Input: part model. Units: mm. Frame: model coordinates. A direction names the side the tool comes from. Coordinates: 2 decimals unless noted, no trailing zeros. Loops run counter-clockwise (first coordinate to the right, second up) from the corner with the lowest first, then second, coordinate; pieces in that order, holes last.
Item 1: Section C-C on z = 5. Return loops of the section in (x, y), and give its area (3 significant figures).
Item 2: Section D-D on z = -1. Give the number of separate pieces and of enclosed holes in the cut face, and give its area (3 significant figures).
Item 3: Reachability of faces 1 (the flat face through (-3, 8, -6)), 2 (the cylindrical face through (-7.8, -5.42, 5.42)), 3 (the cylindrical face through (-2.422, 3.075, -2.168)), 4 (the cylindrical face through (0.3, 3.4, 3.1)) from +Z, -Z, +X, -X, +Y, -Y: full face, straight path, thin tool, end or side. Return the list, or none.
Item 4: Contact query for flat-ended pins moving along their axis: P1, Ø10, axis at x = 1, y = -0.5, coming from the +Z side; P2, Ø3.5, axis at x = 12, y = 12, coming from the -Z side; P3, Ø1.2, axis at y = 8, z = -6, coming from the +X side. Output: stop coordinate, or through.
Item 5: Section B-B on y = 11. Return loops of the section in (x, z).
Item 6: Ray query, line 1 along Y through (x, z) = (0, -2.25); line 2 along Y through (x, z) = (0, 3.1); line 3 along X through (y, z) = (-6, -1). Return the intervals inside material, ascending.
Item 7: Section A-A on x = -12. Return loops of the section in (y, z).
Autodesk Inventor part; units mm, degrees
ref_plane "YZ Plane" through (0, 0, 0) normal (1, 0, 0) x (0, 1, 0)
ref_plane "XZ Plane" through (0, 0, 0) normal (0, 1, 0) x (-1, 0, 0)
ref_plane "XY Plane" through (0, 0, 0) normal (0, 0, 1) x (1, 0, 0)
sketch "Sketch1" plane through (0, 0, 0) normal (0, 0, 1) x (1, 0, 0)
  line L0 (15, 15) -> (-15, 15)
  line L1 (-15, 15) -> (-15, -15)
  line L2 (-15, -15) -> (15, -15)
  line L3 (15, -15) -> (15, 15)
  point P0 (0, 0)
  point P1 (15, 0)
  point P2 (0, 15)
  dimension "d0" = 30
extrude "Extrusion1" add sketch "Sketch1" along normal blind 2.3876
fillet "Fillet1" radius 5 4 edges at (15, 15, 1.1938) (-15, 15, 1.1938) (-15, -15, 1.1938) (15, -15, 1.1938)
sketch "Sketch2" plane through (0, 0, 2.3876) normal (0, 0, 1) x (1, 0, 0)
  line L0 (10, -15) -> (-10, -15)
  line L1 (15, 10) -> (15, -10)
  line L2 (-10, 15) -> (10, 15)
  line L3 (-15, -10) -> (-15, 10)
  point P0 (-12, 12)
  point P1 (12, 12)
  point P2 (12, -12)
  point P3 (-12, -12)
  dimension "d4" = 3
  dimension "d5" = 3
  dimension "d6" = 3
  dimension "d7" = 3
hole "Hole1" at (-12, 12, 2.3876) at (12, 12, 2.3876) at (12, -12, 2.3876) at (-12, -12, 2.3876) direction (0, 0, -1) diameter 3 end through all
sketch "Sketch3" plane through (0, 0, 2.3876) normal (0, 0, 1) x (1, 0, 0)
  line L0 (15, 10) -> (15, -10)
  line L1 (-10, 15) -> (10, 15)
  circle A0 centre (0, 0) radius 12.5
  point P0 (15, 0)
  point P1 (0, 15)
  dimension "d15" = 25
extrude "Extrusion2" add sketch "Sketch3" along normal blind 5
sketch "Sketch4" plane through (0, 0, 7.3876) normal (0, 0, 1) x (1, 0, 0)
  circle A0 centre (0, 0) radius 12.5
  circle A1 centre (0, 0) radius 9.5
  dimension "d86" = 3
extrude "Extrusion3" cut sketch "Sketch4" against normal blind 4 contours A1
sketch "Sketch5" plane through (0, 0, 7.3876) normal (0, 0, 1) x (1, 0, 0)
  circle A0 centre (0, 0) radius 9.5
  circle A1 centre (0, 0) radius 12.5
  circle A2 centre (0, 0) radius 10.5
  line L0 (-2, 9.2871) -> (-2, 10.3078)
  line L1 (2, 9.2871) -> (2, 10.3078)
  dimension "d23" = 4
  dimension "d85" = 2
extrude "Extrusion4" cut sketch "Sketch5" against normal up to surface (4 mm away) contours A0 L0 A2 L1 picked at (-1.557, 9.6904)
sketch "Sketch6" plane through (0, 0, 7.3876) normal (0, 0, 1) x (1, 0, 0)
  line L0 (2, 10.3078) -> (2, 9.2871)
  arc A0 (-2, 9.2871) -> (2, 9.2871) centre (0, 0) ccw
  line L1 (-2, 9.2871) -> (-2, 10.3078)
  arc A1 (2, 10.3078) -> (-2, 10.3078) centre (0, 0) ccw
  circle A2 centre (0, 0) radius 12.5
  circle A3 centre (0, 0) radius 10.5
  line L2 (-9.3841, -1.4792) -> (-10.3549, -1.7393)
  line L3 (-8.8665, -3.411) -> (-9.8373, -3.6712)
  line L4 (-6.2379, -7.1651) -> (-6.8143, -7.9884)
  line L5 (-5.176, -9.1356) -> (-4.5996, -8.3123)
  line L6 (4.5996, -8.3123) -> (5.176, -9.1356)
  line L7 (6.2379, -7.1651) -> (6.8143, -7.9884)
  line L8 (9.4984, 0.1728) -> (10.4997, 0.0852)
  line L9 (9.3241, -1.8196) -> (10.3253, -1.9072)
  dimension "d26" = 105
  dimension "d27" = 2
  dimension "d30" = 2
  dimension "d31" = 40
  dimension "d32" = 70
  dimension "d33" = 2
  dimension "d34" = 2
  dimension "d35" = 50
extrude "Extrusion5" cut sketch "Sketch6" against normal up to surface (4 mm away) contours L0 A0 L1 A1 | A3 L9 A0 L8 | L2 A0 L3 A3 | L7 A3 L6 A0 | L4 A0 L5 A3
sketch "Sketch7" plane through (0, 0, 3.3876) normal (0, 0, 1) x (1, 0, 0)
  arc A0 (2, 10.3078) -> (-2, 10.3078) centre (0, 0) ccw
  circle A1 centre (0, 0) radius 8
  arc A2 (-2, 9.2871) -> (-9.3841, -1.4792) centre (0, 0) ccw
  dimension "d84" = 1.5
extrude "Extrusion6" add sketch "Sketch7" along normal blind 0.381
sketch "Sketch8" plane through (0, 0, 0) normal (0, 0, -1) x (-1, 0, 0)
  line L0 (-10, 15) -> (10, 15)
  line L1 (-15, -10) -> (-15, 10)
  circle A0 centre (0, 0) radius 10
  point P0 (-15, 0)
  point P1 (0, 15)
  dimension "d39" = 20
extrude "Extrusion7" add sketch "Sketch8" along normal blind 5.715
sketch "Sketch9" plane through (0, 0, -5.715) normal (0, 0, -1) x (-1, 0, 0)
  circle A0 centre (0, 0) radius 10
  circle A1 centre (0, 0) radius 9
  dimension "d83" = 1
extrude "Extrusion8" add sketch "Sketch9" along normal blind 1.27 contours A1
sketch "Sketch10" plane through (0, 0, -6.985) normal (0, 0, -1) x (-1, 0, 0)
  circle A0 centre (0, 0) radius 9
  circle A1 centre (0, 0) radius 8
  line L0 (-3, 7.4162) -> (-3, 8.4853)
  line L1 (3, 7.4162) -> (3, 8.4853)
  dimension "d46" = 6
  dimension "d82" = 1
extrude "Extrusion9" cut sketch "Sketch10" against normal up to surface (1.27 mm away) contours L1 A1 L0 A0 picked at (-1.8485, 8.4268)
sketch "Sketch11" plane through (0, 0, 3.7686) normal (0, 0, 1) x (1, 0, 0)
  circle A0 centre (0, 0) radius 8
  line L0 (0, 0) -> (0, 6) construction
  point P0 (0, 3)
  point P1 (-2.1213, 2.1213)
  point P2 (-3, 0)
  point P3 (-2.1213, -2.1213)
  point P4 (0, -3)
  point P5 (2.1213, -2.1213)
  point P6 (3, 0)
  point P7 (2.1213, 2.1213)
  point P8 (4.2426, 4.2426)
  point P9 (6, 0)
  point P10 (4.2426, -4.2426)
  point P11 (0, -6)
  point P12 (-4.2426, -4.2426)
  point P13 (-6, 0)
  point P14 (-4.2426, 4.2426)
  dimension "d49" = 3
  dimension "d52" = 360
  dimension "d87" = 6
  dimension "d90" = 360
hole "Hole2" at (0, 0, 3.7686) at (0, 3, 3.7686) at (-2.1213, 2.1213, 3.7686) at (-3, 0, 3.7686) at (-2.1213, -2.1213, 3.7686) at (0, -3, 3.7686) at (2.1213, -2.1213, 3.7686) at (3, 0, 3.7686) at (2.1213, 2.1213, 3.7686) at (0, 6, 3.7686) at (4.2426, 4.2426, 3.7686) at (6, 0, 3.7686) at (4.2426, -4.2426, 3.7686) at (0, -6, 3.7686) at (-4.2426, -4.2426, 3.7686) at (-6, 0, 3.7686) at (-4.2426, 4.2426, 3.7686) direction (0, 0, -1) diameter 1 end through all
sketch "Sketch12" plane through (0, 0, -6.985) normal (0, 0, -1) x (-1, 0, 0)
  circle A0 centre (-3, 0) radius 0.5
  circle A1 centre (0, -3) radius 0.5
  circle A2 centre (3, 0) radius 0.5
  circle A3 centre (0, 3) radius 0.5
  circle A4 centre (0, 0) radius 0.5
  circle A5 centre (2.1213, 2.1213) radius 0.5
  circle A6 centre (2.1213, -2.1213) radius 0.5
  circle A7 centre (-2.1213, -2.1213) radius 0.5
  circle A8 centre (-2.1213, 2.1213) radius 0.5
  point P0 (6, 0)
  point P1 (0, -6)
  point P2 (-6, 0)
  point P3 (0, 6)
  point P4 (-4.2426, 4.2426)
  point P5 (-4.2426, -4.2426)
  point P6 (4.2426, -4.2426)
  point P7 (4.2426, 4.2426)
  point P8 (0, 0)
  point P9 (0, 0)
hole "Hole3" at (0, 3, -6.985) at (2.1213, 2.1213, -6.985) at (3, 0, -6.985) at (2.1213, -2.1213, -6.985) at (0, 0, -6.985) at (-2.1213, 2.1213, -6.985) at (-3, 0, -6.985) at (-2.1213, -2.1213, -6.985) at (0, -3, -6.985) at (4.2426, 4.2426, -6.985) at (0, 6, -6.985) at (-4.2426, 4.2426, -6.985) at (-6, 0, -6.985) at (-4.2426, -4.2426, -6.985) at (0, -6, -6.985) at (4.2426, -4.2426, -6.985) at (6, 0, -6.985) direction (0, 0, 1) diameter 2 depth 9.5
sketch "Sketch13" plane through (0, 0, -6.985) normal (0, 0, -1) x (-1, 0, 0)
  arc A0 (-3, 8.4853) -> (3, 8.4853) centre (0, 0) ccw
  line L0 (3, 8.4853) -> (3, 7.4162)
  arc A1 (3, 7.4162) -> (-3, 7.4162) centre (0, 0) ccw
  circle A2 centre (0, 0) radius 8
  line L1 (-2.5, -8.6458) -> (-2.5, -7.5993)
  line L2 (2.5, -8.6458) -> (2.5, -7.5993)
  dimension "d68" = 5
extrude "Extrusion10" cut sketch "Sketch13" against normal up to surface (1.27 mm away) contours L1 A2 L2 A0
sketch "Sketch25" plane through (0, 0, 3.7686) normal (0, 0, 1) x (1, 0, 0)
  line L0 (-1.0163, 4.6819) -> (0.1279, 4.6819) construction
  line L1 (0.1279, 4.6819) -> (0.1279, 3.2031) construction
  line L2 (0.1279, 3.2031) -> (-1.0163, 3.2031) construction
  line L3 (-1.0163, 3.2031) -> (-1.0163, 4.6819) construction
  line L4 (3.2538, -0.055) -> (3.2538, 1.4238) construction
  line L5 (3.2538, 1.4238) -> (4.398, 1.4238) construction
  line L6 (4.398, 1.4238) -> (4.398, -0.055) construction
  line L7 (4.398, -0.055) -> (3.2538, -0.055) construction
  line L8 (1.6906, 2.4904) -> (1.6906, 3.9692) construction
  line L9 (1.6906, 3.9692) -> (2.8348, 3.9692) construction
  line L10 (2.8348, 3.9692) -> (2.8348, 2.4904) construction
  line L11 (2.8348, 2.4904) -> (1.6906, 2.4904) construction
  line L12 (-2.7944, -4.281) -> (-2.7944, -2.8021) construction
  line L13 (-2.7944, -2.8021) -> (-1.6502, -2.8021) construction
  line L14 (-1.6502, -2.8021) -> (-1.6502, -4.281) construction
  line L15 (-1.6502, -4.281) -> (-2.7944, -4.281) construction
  line L16 (-3.4049, 1.9851) -> (-3.4049, 3.4639) construction
  line L17 (-3.4049, 3.4639) -> (-2.2607, 3.4639) construction
  line L18 (-2.2607, 3.4639) -> (-2.2607, 1.9851) construction
  line L19 (-2.2607, 1.9851) -> (-3.4049, 1.9851) construction
  line L20 (-0.3938, -2.1662) -> (-0.3938, -0.6874) construction
  line L21 (-0.3938, -0.6874) -> (0.7504, -0.6874) construction
  line L22 (0.7504, -0.6874) -> (0.7504, -2.1662) construction
  line L23 (0.7504, -2.1662) -> (-0.3938, -2.1662) construction
  line L24 (0.0431, -4.9913) -> (0.0431, -3.5125) construction
  line L25 (0.0431, -3.5125) -> (1.1873, -3.5125) construction
  line L26 (1.1873, -3.5125) -> (1.1873, -4.9913) construction
  line L27 (1.1873, -4.9913) -> (0.0431, -4.9913) construction
  line L28 (-4.4721, -0.8803) -> (-4.4721, 0.5985) construction
  line L29 (-4.4721, 0.5985) -> (-3.3279, 0.5985) construction
  line L30 (-3.3279, 0.5985) -> (-3.3279, -0.8803) construction
  line L31 (-3.3279, -0.8803) -> (-4.4721, -0.8803) construction
  line L32 (-0.7955, 6.2805) -> (-0.7955, 7.7593) construction
  line L33 (-0.7955, 7.7593) -> (0.3487, 7.7593) construction
  line L34 (0.3487, 7.7593) -> (0.3487, 6.2805) construction
  line L35 (0.3487, 6.2805) -> (-0.7955, 6.2805) construction
  line L36 (2.6912, -3.4816) -> (2.6912, -2.0028) construction
  line L37 (2.6912, -2.0028) -> (3.8354, -2.0028) construction
  line L38 (3.8354, -2.0028) -> (3.8354, -3.4816) construction
  line L39 (3.8354, -3.4816) -> (2.6912, -3.4816) construction
  line L40 (6.0179, 0.2278) -> (6.0179, 1.7067) construction
  line L41 (6.0179, 1.7067) -> (7.1621, 1.7067) construction
  line L42 (7.1621, 1.7067) -> (7.1621, 0.2278) construction
  line L43 (7.1621, 0.2278) -> (6.0179, 0.2278) construction
  line L44 (3.4493, 4.5372) -> (3.4493, 6.016) construction
  line L45 (3.4493, 6.016) -> (4.5935, 6.016) construction
  line L46 (4.5935, 6.016) -> (4.5935, 4.5372) construction
  line L47 (4.5935, 4.5372) -> (3.4493, 4.5372) construction
  line L48 (3.4493, -6.362) -> (3.4493, -4.8831) construction
  line L49 (3.4493, -4.8831) -> (4.5935, -4.8831) construction
  line L50 (4.5935, -4.8831) -> (4.5935, -6.362) construction
  line L51 (4.5935, -6.362) -> (3.4493, -6.362) construction
  line L52 (-1.904, -8) -> (-1.904, -6.5212) construction
  line L53 (-1.904, -6.5212) -> (-0.7598, -6.5212) construction
  line L54 (-0.7598, -6.5212) -> (-0.7598, -8) construction
  line L55 (-0.7598, -8) -> (-1.904, -8) construction
  line L56 (-6.5, -4.8831) -> (-6.5, -3.4043) construction
  line L57 (-6.5, -3.4043) -> (-5.3558, -3.4043) construction
  line L58 (-5.3558, -3.4043) -> (-5.3558, -4.8831) construction
  line L59 (-5.3558, -4.8831) -> (-6.5, -4.8831) construction
  line L60 (-7.769, 0.2278) -> (-7.769, 1.7067) construction
  line L61 (-7.769, 1.7067) -> (-6.6248, 1.7067) construction
  line L62 (-6.6248, 1.7067) -> (-6.6248, 0.2278) construction
  line L63 (-6.6248, 0.2278) -> (-7.769, 0.2278) construction
  line L64 (-4.7426, 4.7426) -> (-4.7426, 6.2215) construction
  line L65 (-4.7426, 6.2215) -> (-3.5984, 6.2215) construction
  line L66 (-3.5984, 6.2215) -> (-3.5984, 4.7426) construction
  line L67 (-3.5984, 4.7426) -> (-4.7426, 4.7426) construction
ref_plane "Work Plane2" through (0, 0, -12.985) normal (0, 0, -1) x (-1, 0, 0)
ref_plane "Work Plane3" through (0, 0, -14.985) normal (0, 0, -1) x (-1, 0, 0)
equation "\"d30\" = d27"
equation "\"d33\" = d30"
equation "\"d34\" = d33"
properties part number "3601243"
Results found:
1. outline: circle Ø25 at (0, 0); hole (-10.35, -1.74) arc R10.5 ccw to (-9.84, -3.67) - (-8.87, -3.41) arc R9.5 ccw to (-6.24, -7.17) - (-6.81, -7.99) arc R10.5 ccw to (-5.18, -9.14) - (-4.6, -8.31) arc R9.5 ccw to (4.6, -8.31) - (5.18, -9.14) arc R10.5 ccw to (6.81, -7.99) - (6.24, -7.17) arc R9.5 ccw to (9.32, -1.82) - (10.33, -1.91) arc R10.5 ccw to (10.5, 0.09) - (9.5, 0.17) arc R9.5 ccw to (2, 9.29) - (2, 10.31) arc R10.5 ccw to (-2, 10.31) - (-2, 9.29) arc R9.5 ccw to (-9.38, -1.48) - close
1. area: 195 mm2
2. separate pieces: 1
2. enclosed holes: 17
2. area: 261 mm2
3. face 1: -Z, +Y
3. face 2: +Z
3. face 3: -Z
3. face 4: +Z, -Z
4. P1: stops at z = 3.77
4. P2: stops at z = 0
4. P3: stops at x = 6.65
5. outline: (-14.9, 0) - (-13.12, 0) - (-13.12, 2.39) - (-14.9, 2.39) - close; (-10.88, 0) - (10.88, 0) - (10.88, 2.39) - (5.94, 2.39) - (5.94, 7.39) - (-5.94, 7.39) - (-5.94, 2.39) - (-10.88, 2.39) - close; (13.12, 0) - (14.9, 0) - (14.9, 2.39) - (13.12, 2.39) - close
6. line 1: y = -10 to -7, -5 to -4, -2 to -1, 1 to 2, 4 to 5, 7 to 10
6. line 2: y = -12.5 to -6.5, -5.5 to -3.5, -2.5 to -0.5, 0.5 to 2.5, 3.5 to 5.5, 6.5 to 12.5
6. line 3: x = -8 to -1, 1 to 8
7. outline: (-14.58, 0) - (-13.5, 0) - (-13.5, 2.39) - (-14.58, 2.39) - close; (-10.5, 0) - (10.5, 0) - (10.5, 2.39) - (3.5, 2.39) - (3.5, 7.39) - (-3.5, 7.39) - (-3.5, 2.39) - (-10.5, 2.39) - close; (13.5, 0) - (14.58, 0) - (14.58, 2.39) - (13.5, 2.39) - close
